Drawing for the job (mm, zero at the part's lowest x, y, z). Give positions to 0.01 mm unless a question says otherwise; leave off trailing zeros. Write each loop counter-clockwise with the first axis right and the second up, starting at its lowest first coordinate (ties: lowest second). Pieces come first, ordered by that corner, then holes. Notation, with made-up numbers: M 72.25,57.25 L 79.25,57.25 A12 cw 79.25,62.25 Z; hole C -15,19 d4. An arc over 180 degrees is marked long. Use CSV: the item, a comma, the result in double quotes. Start each with the question number.
1. Drop flat-ended pins along their axis: pin 1 Ø8 at (y, z) = (8.5, 47.5) entering from +X; pin 2 Ø10 at (y, z) = (12.5, 16) entering from -X. Give the stop position or say it passes through.
2. Drill centre lines: line 1 along X through (y, z) = (12.5, 74); line 2 along X through (y, z) = (5.5, 32). Where is each one in solid material? Low to high. Write a range as from..to.
3. Band-saw the part on A-A, the plane y = 15.5. List the corners of the cut face in (x, z) (1 decimal), then the cut area to 3 significant figures.
4. Band-saw the part on C-C, the plane z = 17.5. List the corners of the cut face in (x, y), then the cut area to 3 significant figures.
5. Band-saw the part on B-B, the plane z = 98.5. List the corners of the cut face in (x, y), then the cut area to 3 significant figures.
6. Band-saw the part on D-D, the plane z = 122. List the corners of the cut face in (x, y).
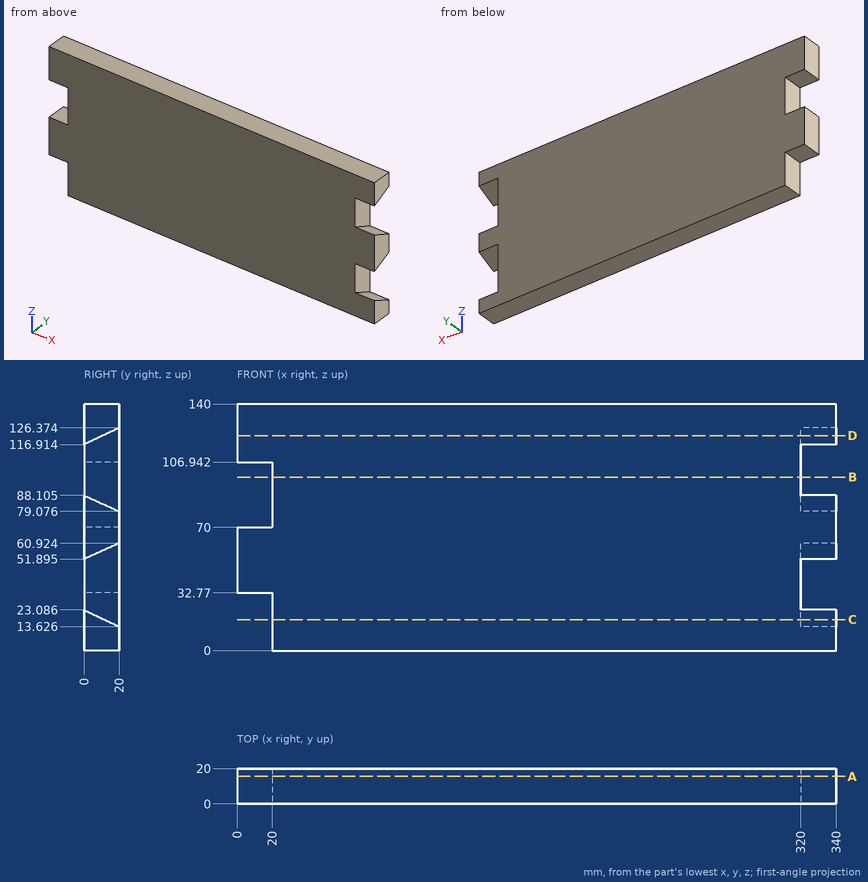
Output:
1,pin 1,"stops at x = 320"
1,pin 2,"stops at x = 20"
2,line 1,"x = 20..340"
2,line 2,"x = 20..320"
3,outline,"M 0,32.8 L 20,32.8 L 20,0 L 340,0 L 340,15.8 L 320,15.8 L 320,58.9 L 340,58.9 L 340,81.1 L 320,81.1 L 320,124.2 L 340,124.2 L 340,140 L 0,140 L 0,106.9 L 20,106.9 L 20,70 L 0,70 Z"
3,area,"44,500 mm²"
4,outline,"M 20,0 L 340,0 L 340,11.81 L 320,11.81 L 320,20 L 20,20 Z"
4,area,"6,240 mm²"
5,outline,"M 20,0 L 320,0 L 320,20 L 20,20 Z"
5,area,"6,000 mm²"
6,outline,"M 0,0 L 340,0 L 340,10.75 L 320,10.75 L 320,20 L 0,20 Z"
